from build123d import *

# Parameters (mm, degrees)
ESQUISSE1_W             = 200
ESQUISSE1_H             = 160
BOSS_EXTRU_1_DEPTH      = 230
CONG_1_R                = 10
ESQUISSE2_W             = 170
ESQUISSE2_H             = 200
ENL_V_MAT_EXTRU_1_DEPTH = 20
ESQUISSE3_W             = 15
ESQUISSE3_H             = 21
ENL_V_MAT_EXTRU_2_DEPTH = 18
CONG_2_R                = 10
CONG_3_R                = 10
ESQUISSE6_W             = 180
ESQUISSE6_H             = 124
ENL_V_MAT_EXTRU_4_DEPTH = 130
ESQUISSE7_W             = 180
ESQUISSE7_H             = 2
ENL_V_MAT_EXTRU_5_DEPTH = 2
CONG_5_R                = 10
ESQUISSE8_R             = 6.5
ENL_V_MAT_EXTRU_6_DEPTH = 15
ESQUISSE9_W             = 100
ESQUISSE9_H             = 55
ENL_V_MAT_EXTRU_7_DEPTH = 10


with BuildPart() as part:
    # Esquisse1 → Boss.-Extru.1 (new body)
    with BuildSketch(Plane.XY):
        with Locations((100, 80)):
            Rectangle(ESQUISSE1_W, ESQUISSE1_H)
    extrude(amount=BOSS_EXTRU_1_DEPTH)

    # Congé1
    cong_1_edges = [part.edges().sort_by_distance(p)[0] for p in [
        (200, 80, 230),
        (0, 80, 230),
        (200, 80, 0),
        (0, 80, 0),
    ]]
    fillet(cong_1_edges, radius=CONG_1_R)

    # Esquisse2 → Enlèv. mat.-Extru.1 (cut)
    with BuildSketch(Plane.XZ):
        with Locations((100, 115)):
            Rectangle(ESQUISSE2_W, ESQUISSE2_H)
    extrude(amount=-ENL_V_MAT_EXTRU_1_DEPTH, mode=Mode.SUBTRACT)

    # Esquisse3 → Enlèv. mat.-Extru.2 (cut)
    with BuildSketch(Plane(origin=(0, 0, 0), x_dir=(-1, 0, 0), z_dir=(0, -1, 0))):
        with Locations((-7.5, -45.013282715)):
            Rectangle(ESQUISSE3_W, ESQUISSE3_H)
        with Locations((-192.5, -45.013282715)):
            Rectangle(ESQUISSE3_W, ESQUISSE3_H)
        with Locations((-192.5, -184.986717285)):
            Rectangle(ESQUISSE3_W, ESQUISSE3_H)
        with Locations((-7.5, -184.986717285)):
            Rectangle(ESQUISSE3_W, ESQUISSE3_H)
    extrude(amount=-ENL_V_MAT_EXTRU_2_DEPTH, mode=Mode.SUBTRACT)

    # Congé2
    cong_2_edges = [part.edges().sort_by_distance(p)[0] for p in [
        (192.5, 18, 34.513282715),
        (192.5, 18, 55.513282715),
    ]]
    fillet(cong_2_edges, radius=CONG_2_R)

    # Congé3
    cong_3_edges = [part.edges().sort_by_distance(p)[0] for p in [
        (7.5, 18, 34.513282715),
        (7.5, 18, 55.513282715),
    ]]
    fillet(cong_3_edges, radius=CONG_3_R)

    # Esquisse6 → Enlèv. mat.-Extru.4 (cut)
    with BuildSketch(Plane(origin=(0, 0, 0), x_dir=(-1, 0, 0), z_dir=(0, 0, -1))):
        with Locations((-100, 96)):
            Rectangle(ESQUISSE6_W, ESQUISSE6_H)
    extrude(amount=-ENL_V_MAT_EXTRU_4_DEPTH, mode=Mode.SUBTRACT)

    # Esquisse7 → Enlèv. mat.-Extru.5 (cut)
    with BuildSketch(Plane(origin=(0, 0, 0), x_dir=(-1, 0, 0), z_dir=(0, 0, -1))):
        with Locations((-100, 159)):
            Rectangle(ESQUISSE7_W, ESQUISSE7_H)
    extrude(amount=-ENL_V_MAT_EXTRU_5_DEPTH, mode=Mode.SUBTRACT)

    # Congé5
    cong_5_edges = [part.edges().sort_by_distance(p)[0] for p in [
        (7.5, 18, 195.486717285),
        (7.5, 18, 174.486717285),
        (192.5, 18, 195.486717285),
        (192.5, 18, 174.486717285),
    ]]
    fillet(cong_5_edges, radius=CONG_5_R)

    # Esquisse8 → Enlèv. mat.-Extru.6 (cut)
    with BuildSketch(Plane.XY.offset(230)):
        with Locations((100.086517688, 127.081087589)):
            Circle(ESQUISSE8_R)
    extrude(amount=-ENL_V_MAT_EXTRU_6_DEPTH, mode=Mode.SUBTRACT)

    # Esquisse9 → Enlèv. mat.-Extru.7 (cut)
    with BuildSketch(Plane.XY.offset(230)):
        with Locations((100.086517688, 77.5)):
            Rectangle(ESQUISSE9_W, ESQUISSE9_H)
    extrude(amount=-ENL_V_MAT_EXTRU_7_DEPTH, mode=Mode.SUBTRACT)


solid = part.part
For this review, take the finished solid that the model builds, in its own axes (mm). A direction names the side the tool comes from. Coordinates: 2 decimals unless noted, no trailing zeros. Loops run counter-clockwise (first coordinate to the right, second up) from the corner with the lowest first, then second, coordinate; pieces in that order, holes last. Notation, with made-up numbers: (89.25, 33) - (112.25, 33) arc R17 cw to (112.25, 55) - close; hole circle Ø1 at (-32, 74.5). An arc over 180 degrees is marked (long way). Use a Markdown table: item, result. Add a question column.
Item 1: Insertion check: pin 1 Ø8 at (x, z) = (135.5, 116) entering from -Y; pin 2 Ø4 at (x, y) = (6, 5.5) entering from +Z; pin 3 Ø4 at (x, y) = (57.5, 75) entering from +Z. Each pin has a flat end and moves straight along its axis. Give the tip position at first contact, or say it passes through.
Item 2: We need section C-C (y = 116). Give the boundary of the cut face in (x, z), and give its area (3 significant figures).
Item 3: For line 1 (Z direction, x = 154.5, y = 10.5); line 2 (Y direction, x = 22.5, z = 46.5); line 3 (X direction, y = 13.5, z = 18), list the stretches that pass through material, from the lowest coordinate up.
Item 4: Tool access review of faces 1 (the face through (190, 96, 64)), 2 (the face through (7.4, 15.15, 192.48)), 3 (the face through (15, 10, 114)): name each direction out of +Z, -Z, +X, -X, +Y, -Y from which nothing blocks a thin tool from reaching the whole face with its end or side.
Item 5: We need section B-B (x = 144). Give the boundary of the cut face in (y, z), and give its area (3 significant figures).
Item 6: We need section A-A (z = 21). Give the boundary of the cut face in (x, y).
Item 7: We need section D-D (y = 14.5). Give the boundary of the cut face in (x, z), and give its area (3 significant figures).
Item 8: Mouldability with a two-part tool opening along Y and no side actions: class faces 4 (the face through (192.4, 14.99, 37.36)), 5 (the face through (99, 10, 15)), 6 (the face through (101, 158, 65)) as pulls with the +Y half, pulls with the -Y half, needs draft (parallel to the pull), parting line crosses it, or undercut.
Results list:
| question | item | result |
|---|---|---|
| 1 | pin 1 | stops at y = 20 |
| 1 | pin 2 | stops at z = 229.8 |
| 1 | pin 3 | stops at z = 220 |
| 2 | outline | (0, 10) arc R10 ccw to (10, 0) - (10, 130) - (190, 130) - (190, 0) arc R10 ccw to (200, 10) - (200, 220) arc R10 ccw to (190, 230) - (10, 230) arc R10 ccw to (0, 220) - close |
| 2 | area | 22,500 mm^2 |
| 3 | line 1 | z = 0 to 15, 215 to 230 |
| 3 | line 2 | y = 20 to 34, 158 to 160 |
| 3 | line 3 | x = 0 to 15, 185 to 200 |
| 4 | face 1 | -Z |
| 4 | face 2 | +X, -X, -Y |
| 4 | face 3 | -Y |
| 5 | outline | (0, 0) - (34, 0) - (34, 130) - (158, 130) - (158, 2) - (160, 2) - (160, 230) - (105, 230) - (105, 220) - (50, 220) - (50, 230) - (0, 230) - (0, 215) - (20, 215) - (20, 15) - (0, 15) - close |
| 5 | area | 16,100 mm^2 |
| 6 | outline | (0, 0) - (15, 0) - (15, 20) - (185, 20) - (185, 0) - (200, 0) - (200, 160) - (0, 160) - close; hole (10, 34) - (190, 34) - (190, 158) - (10, 158) - close |
| 7 | outline | (0, 10) arc R10 ccw to (10, 0) - (190, 0) arc R10 ccw to (200, 10) - (200, 36.91) - (185, 36.91) - (185, 15) - (15, 15) - (15, 36.91) - (0, 36.91) - close; (0, 53.11) - (15, 53.11) - (15, 176.89) - (0, 176.89) - close; (0, 193.09) - (15, 193.09) - (15, 215) - (185, 215) - (185, 193.09) - (200, 193.09) - (200, 220) arc R10 ccw to (190, 230) - (10, 230) arc R10 ccw to (0, 220) - close; (185, 53.11) - (200, 53.11) - (200, 176.89) - (185, 176.89) - close |
| 7 | area | 10,900 mm^2 |
| 8 | face 4 | pulls with the -Y half |
| 8 | face 5 | needs draft |
| 8 | face 6 | undercut |
